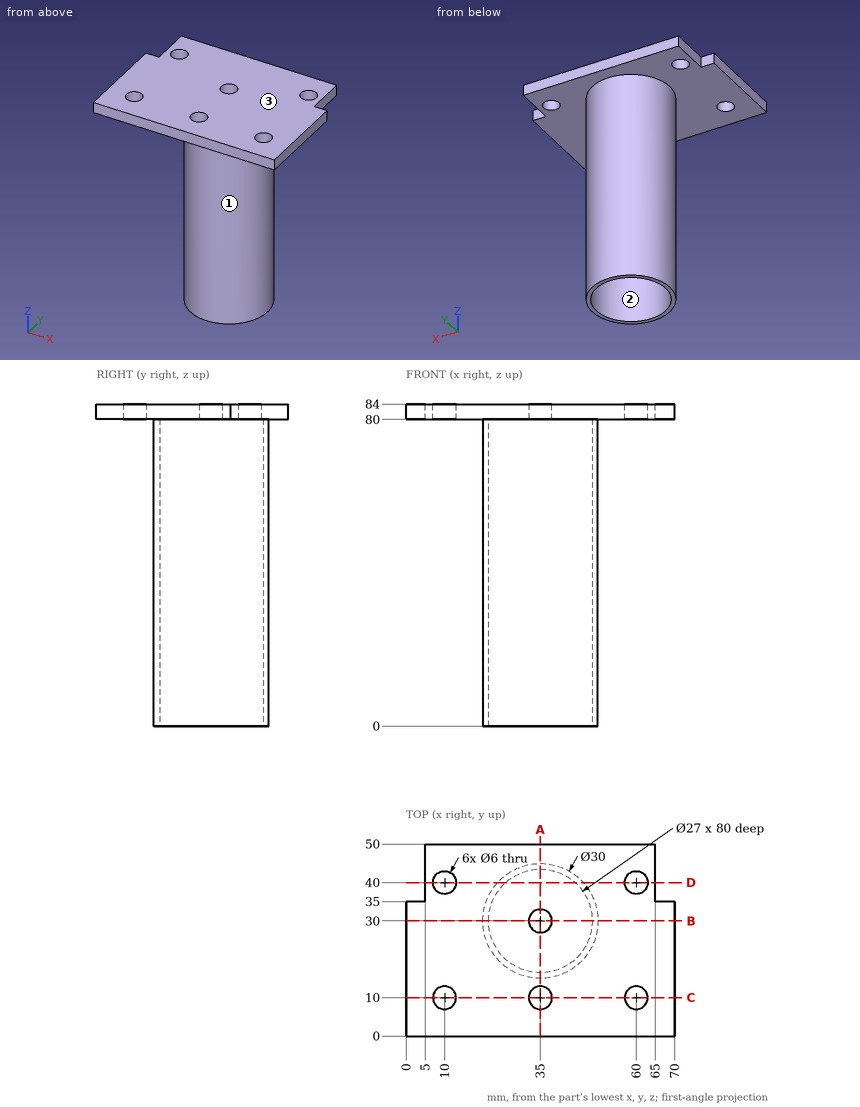
Geometry check sheet. Reference: drawing and pictorial views, mm from the part's lowest x, y, z. Round coordinates to 2 decimals unless told otherwise and drop trailing zeros. Order: outer loops, then holes, each group sorted by start corner. A loop starts at its lowest first (then second) coordinate and runs counter-clockwise, first axis right, second up. Notation, with made-up numbers: M 85,56.25 L 100,56.25 A30 cw 100,85.25 Z; hole C 21,37.25 d7. An arc over 180 degrees is marked long. One line per item, written item: value. Start each with the question number.
1. Section check A-A on x = 35. Enter the section's corners in (y, z), and give its area (3 significant figures).
2. Section check B-B on y = 30. Enter the section's corners in (x, z).
3. Gauge pin test, flat ends, axial feed: P1, Ø2, axis at x = 25.5, z = 10.5, coming from the -Y side; P2, Ø9.5, axis at x = 10, y = 40, coming from the -Z side; P3, Ø2, axis at x = 66.5, z = 81.5, coming from the +Y side. Record the tip position at first contact, or that the pin passes through.
4. Release check for a two-part mould opening along Y. For the marked faces 1, 2 and 3 record: released by +Y, released by -Y, zero draft, split by the parting line, or undercut.
5. Scan lines: line 1 along Y through (x, z) = (10, 83); line 2 along Z through (x, y) = (51, 43); line 3 along Y through (x, z) = (36.5, 73). Record each from-to range of solid material in increasing order.
6. Section check D-D on y = 40. Enter the section's corners in (x, z), and give its area (3 significant figures).
7. Section check C-C on y = 10. Enter the section's corners in (x, z), and give its area (3 significant figures).
Results found:
1. outline: M 0,80 L 7,80 L 7,84 L 0,84 Z; M 13,80 L 15,80 L 15,0 L 16.5,0 L 16.5,80 L 27,80 L 27,84 L 13,84 Z; M 33,80 L 43.5,80 L 43.5,0 L 45,0 L 45,80 L 50,80 L 50,84 L 33,84 Z
1. area: 392 mm^2
2. outline: M 0,80 L 20,80 L 20,0 L 21.5,0 L 21.5,80 L 32,80 L 32,84 L 0,84 Z; M 38,80 L 48.5,80 L 48.5,0 L 50,0 L 50,80 L 70,80 L 70,84 L 38,84 Z
3. P1: y = 17.64
3. P2: z = 80
3. P3: y = 35
4. face 1: split by the parting line
4. face 2: undercut
4. face 3: zero draft
5. line 1: 0 to 7, 13 to 37, 43 to 50
5. line 2: 80 to 84
5. line 3: 15.08 to 16.58, 43.42 to 44.92
6. outline: M 5,80 L 7,80 L 7,84 L 5,84 Z; M 13,80 L 23.82,80 L 23.82,0 L 25.93,0 L 25.93,80 L 44.07,80 L 44.07,0 L 46.18,0 L 46.18,80 L 57,80 L 57,84 L 13,84 Z; M 63,80 L 65,80 L 65,84 L 63,84 Z
6. area: 530 mm^2
7. outline: M 0,80 L 7,80 L 7,84 L 0,84 Z; M 13,80 L 32,80 L 32,84 L 13,84 Z; M 38,80 L 57,80 L 57,84 L 38,84 Z; M 63,80 L 70,80 L 70,84 L 63,84 Z
7. area: 208 mm^2
